Part model, mm, in its own coordinate system. A direction names the side the tool comes from. Coordinates: 2 decimals unless noted, no trailing zeros. Write each loop counter-clockwise with the first axis right and the second up, starting at its lowest first coordinate (ties: lowest second). Pieces come first, ordered by that corner, then holes. Notation, with made-up numbers: M 63,69.5 L 121,69.5 A11 cw 121,81.5 Z; hole C 48.25,36 d1. An arc over 180 degrees is marked long. Use a Markdown table: item, result. Add a question column.
Q1. Wall check: L1, parallel to X at y = 2.75, z = 0; L2, parallel to X at y = 12.5, z = -14.5; L3, parallel to Y at x = -12, z = -7.5. Give the ranges that are in metal, low to high. Write a range as from..to.
Q2. Pin check, flat tips, straight feed: pin 1 Ø3.5 at (x, y) = (18.5, 17) entering from -Z; pin 2 Ø10 at (x, z) = (-10, 11.5) entering from +Y; pin 3 Ø3 at (x, y) = (-0.5, 11) entering from +Z. Stop position of each tip, or through.
Q3. Tool access for faces 1 (the flat face through (18, 16, -4)), 2 (the flat face through (4, 8, 18)), 3 (the cylindrical face through (4.66, 4.44, 5.09)), 4 (the flat face through (-4, 8, -18)): list every direction of +Z, -Z, +X, -X, +Y, -Y with a clear straight run to the whole face (end or side of a thin tool).
Q4. Slice it at B-B on y = 17. Write the cut outline in (x, z), then the cut area to 3 significant figures.
Q5. Slice it at D-D on y = 8.5. Write the cut outline in (x, z), then the cut area to 3 significant figures.
Q6. Mould opens along X. For faces 5 (the flat face through (3, 3, 16)), 6 (the cylindrical face through (4.363, 12.042, -0.573)), 7 (the cylindrical face through (19.43, 7.6, -19.4)), 8 (the flat face through (10, 7, -20)) say: released by +X, released by -X, zero draft, split by the parting line, or undercut.
Q7. Slice it at C-C on x = 0. Write the cut outline in (y, z).
Q8. Slice it at A-A on z = 0. Write the cut outline in (x, y).
from build123d import *

# Parameters (mm, degrees)
SKETCH_1_W          = 40
SKETCH_1_H          = 40
EXTRUDE_1_DEPTH     = 15
SKETCH_2_W          = 4
SKETCH_2_H          = 8
EXTRUDE_2_DEPTH     = 3
SKETCH_3_R          = 4.4
CUT_EXTRUDE_1_DEPTH = 16
SKETCH_4_R          = 6.9
CUT_EXTRUDE_2_DEPTH = 9
CUT_EXTRUDE_3_DEPTH = 7
SKETCH_6_R          = 5.2
CUT_EXTRUDE_4_DEPTH = 2
FILLET_1_R          = 2


with BuildPart() as part:
    # Эскиз1 → Бобышка-Вытянуть1 (new body)
    with BuildSketch(Plane(origin=(0, 0, 0), x_dir=(1, 0, 0), z_dir=(0, 1, 0))):
        Rectangle(SKETCH_1_W, SKETCH_1_H)
    extrude(amount=EXTRUDE_1_DEPTH)

    # Эскиз2 → Бобышка-Вытянуть2 (add)
    with BuildSketch(Plane(origin=(0, 15, 0), x_dir=(1, 0, 0), z_dir=(0, 1, 0))):
        with Locations((-18, 0)):
            Rectangle(SKETCH_2_W, SKETCH_2_H)
        with Locations((18, 0)):
            Rectangle(SKETCH_2_W, SKETCH_2_H)
    extrude(amount=EXTRUDE_2_DEPTH)

    # Эскиз3 → Вырез-Вытянуть1 (cut, through all)
    with BuildSketch(Plane(origin=(0, 15, 0), x_dir=(1, 0, 0), z_dir=(0, 1, 0))):
        with Locations(Location((0, 0, 0), (0, 0, 270))):  # turned: the seam where the file's is
            Circle(SKETCH_3_R)
        with BuildLine():
            Line((-3, -20), (-3, -13))
            ThreePointArc((-3, -13), (0, -10), (3, -13))
            Line((3, -13), (3, -20))
            Line((3, -20), (-3, -20))
        make_face()
        with BuildLine():
            Line((3, 13), (3, 20))
            Line((3, 20), (-3, 20))
            Line((-3, 20), (-3, 13))
            ThreePointArc((-3, 13), (0, 10), (3, 13))
        make_face()
    extrude(amount=-CUT_EXTRUDE_1_DEPTH, mode=Mode.SUBTRACT)

    # Эскиз4 → Вырез-Вытянуть2 (cut)
    with BuildSketch(Plane.XZ):
        with Locations(Location((0, 0, 0), (0, 0, 270))):  # turned: the seam where the file's is
            Circle(SKETCH_4_R)
    extrude(amount=-CUT_EXTRUDE_2_DEPTH, mode=Mode.SUBTRACT)

    # Эскиз5 → Вырез-Вытянуть3 (cut)
    with BuildSketch(Plane(origin=(0, 15, 0), x_dir=(1, 0, 0), z_dir=(0, 1, 0))):
        with BuildLine():
            Line((-5.2, -20), (-5.2, -13))
            ThreePointArc((-5.2, -13), (0, -7.8), (5.2, -13))
            Line((5.2, -13), (5.2, -20))
            Line((5.2, -20), (-5.2, -20))
        make_face()
        with BuildLine():
            Line((5.2, 13), (5.2, 20))
            Line((5.2, 20), (-5.2, 20))
            Line((-5.2, 20), (-5.2, 13))
            ThreePointArc((-5.2, 13), (0, 7.8), (5.2, 13))
        make_face()
    extrude(amount=-CUT_EXTRUDE_3_DEPTH, mode=Mode.SUBTRACT)

    # Эскиз6 → Вырез-Вытянуть4 (cut)
    with BuildSketch(Plane(origin=(0, 8, 0), x_dir=(1, 0, 0), z_dir=(0, 1, 0))):
        with Locations((0, -13)):
            Circle(SKETCH_6_R)
        with Locations((0, 13)):
            Circle(SKETCH_6_R)
    extrude(amount=-CUT_EXTRUDE_4_DEPTH, mode=Mode.SUBTRACT)

    # Скругление1
    fillet_1_edges = [part.edges().sort_by_distance(p)[0] for p in [
        (-20, 7.5, -20),
        (20, 7.5, -20),
        (20, 7.5, 20),
        (-20, 7.5, 20),
    ]]
    fillet(fillet_1_edges, radius=FILLET_1_R)


solid = part.part
Recorded:
| question | item | result |
|---|---|---|
| 1 | L1 | -20..-6.9, 6.9..20 |
| 1 | L2 | -20..-5.2, 5.2..20 |
| 1 | L3 | 0..15 |
| 2 | pin 1 | z = -4 |
| 2 | pin 2 | y = 15 |
| 2 | pin 3 | z = 8.2 |
| 3 | face 1 | -Z, +X, -X, +Y |
| 3 | face 2 | +Z, +Y |
| 3 | face 3 | -Y |
| 3 | face 4 | -Z, +Y |
| 4 | outline | M -20,-4 L -16,-4 L -16,4 L -20,4 Z; M 16,-4 L 20,-4 L 20,4 L 16,4 Z |
| 4 | area | 64.0 mm² |
| 5 | outline | M -20,-18 A2 ccw -18,-20 L -5.2,-20 L -5.2,-13 A5.2 cw 5.2,-13 L 5.2,-20 L 18,-20 A2 ccw 20,-18 L 20,18 A2 ccw 18,20 L 5.2,20 L 5.2,13 A5.2 cw -5.2,13 L -5.2,20 L -18,20 A2 ccw -20,18 Z; hole C 0,0 d13.8 |
| 5 | area | 1,220 mm² |
| 6 | face 5 | undercut |
| 6 | face 6 | undercut |
| 6 | face 7 | released by +X |
| 6 | face 8 | zero draft |
| 7 | outline | M 0,-10 L 6,-10 L 6,-7.8 L 15,-7.8 L 15,-4.4 L 9,-4.4 L 9,-6.9 L 0,-6.9 Z; M 0,6.9 L 9,6.9 L 9,4.4 L 15,4.4 L 15,7.8 L 6,7.8 L 6,10 L 0,10 Z |
| 8 | outline | M -20,0 L -6.9,0 L -6.9,9 L -4.4,9 L -4.4,15 L -16,15 L -16,18 L -20,18 Z; M 4.4,9 L 6.9,9 L 6.9,0 L 20,0 L 20,18 L 16,18 L 16,15 L 4.4,15 Z |
